Verification items for the finished model (mm, model axes). A direction names the side the tool comes from. Round coordinates to 2 decimals unless told otherwise and drop trailing zeros. Write each loop counter-clockwise with the first axis right and the second up, starting at its lowest first coordinate (ties: lowest second). Pieces come first, ordered by that corner, then holes. Notation, with made-up numbers: (12.5, -21) - (44.5, -21) arc R19 ccw to (44.5, 3) - close; hole circle Ø10 at (-35, -26). An arc over 180 degrees is marked (long way). Answer as a JSON object with one key per item and string values.
```python
from build123d import *

# Parameters (mm, degrees)
BOSS_EXTRUDE2_DEPTH           = 30
FILLET2_R                     = 10
FILLET3_R                     = 10
TAP_DRILL_FOR_M5_HELICOIL1_D  = 5.2
TAP_DRILL_FOR_M8_HELICOIL4_D  = 8.3
TAP_DRILL_FOR_M12_HELICOIL1_D = 12.5
TAP_DRILL_FOR_M8_TAP1_D       = 6.8
TAP_DRILL_FOR_M8_TAP1_DEPTH   = 25
TAP_DRILL_FOR_M8_TAP1_TIP     = 2.042926105
TAP_DRILL_FOR_M8_TAP2_D       = 6.8
TAP_DRILL_FOR_M8_TAP2_DEPTH   = 25
TAP_DRILL_FOR_M8_TAP2_TIP     = 2.042926105
TAP_DRILL_FOR_M8_TAP4_D       = 6.8
TAP_DRILL_FOR_M8_TAP4_DEPTH   = 25
TAP_DRILL_FOR_M8_TAP4_TIP     = 2.042926105
TAP_DRILL_FOR_M8_TAP5_D       = 6.8
TAP_DRILL_FOR_M8_TAP5_DEPTH   = 25
TAP_DRILL_FOR_M8_TAP5_TIP     = 2.042926105


with BuildPart() as part:
    # Sketch1 → Boss-Extrude2 (new body)
    with BuildSketch(Plane.XY):
        Polygon((0, 0), (370, 0), (370, 300), (185, 485), (0, 485), (0, 300), align=None)
        with BuildLine():
            Line((120, 323.710101352), (250, 323.710101352))
            ThreePointArc((250, 323.710101352), (273.710101352, 300), (250, 276.289898648))
            Line((250, 276.289898648), (120, 276.289898648))
            ThreePointArc((120, 276.289898648), (96.289898648, 300), (120, 323.710101352))
        make_face(mode=Mode.SUBTRACT)
    extrude(amount=BOSS_EXTRUDE2_DEPTH)

    # Fillet2
    fillet2_edges = [part.edges().sort_by_distance(p)[0] for p in [
        (370, 0, 15),
        (0, 0, 15),
    ]]
    fillet(fillet2_edges, radius=FILLET2_R)

    # Fillet3
    fillet3_edges = [part.edges().sort_by_distance(p)[0] for p in [
        (0, 485, 15),
        (185, 485, 15),
        (370, 300, 15),
    ]]
    fillet(fillet3_edges, radius=FILLET3_R)

    # Tap Drill for M5 Helicoil1 (through all)
    with Locations(Plane.XY.offset(30)):
        with Locations((300.970994454, 188.552878957), (181.155657642, 94.366491196), (100.424468133, 123.839782605), (151.041642508, 198.804458578), (260.6053997, 227.63702626), (283.030730119, 70.659713324), (88.89144106, 227.63702626), (165.137564486, 383.973615469), (315.707640159, 272.487687099), (61.981044557, 285.302161624)):
            Hole(TAP_DRILL_FOR_M5_HELICOIL1_D / 2)

    # Tap Drill for M8 Helicoil4 (through all)
    with Locations(Plane.XY.offset(30)):
        with Locations((65.825386914, 51.438001536), (45.322227674, 148.828007929), (236.898621828, 139.857875761), (241.383687912, 373.722035849), (338.132970578, 99.492281006), (223.443423576, 37.982803285), (193.970132168, 225.074131355), (36.992819232, 253.26597531)):
            Hole(TAP_DRILL_FOR_M8_HELICOIL4_D / 2)

    # Tap Drill for M12 Helicoil1 (through all)
    with Locations(Plane.XY.offset(30)):
        with Locations((163.856117033, 153.953797739), (325.318496053, 49.561393209), (128.616312088, 79.629845492), (189.485066084, 423.057762771), (110.676047753, 357.063218966), (97.220849501, 178.301299337), (325.318496053, 229.559197439), (53.19045969, 410.886687746)):
            Hole(TAP_DRILL_FOR_M12_HELICOIL1_D / 2)

    # Tap Drill for M8 Tap1
    with Locations(Plane(origin=(0, 0, 0), x_dir=(-1, 0, 0), z_dir=(0, -1, 0))):
        with Locations((-65, -15), (-315, -15)):
            Hole(TAP_DRILL_FOR_M8_TAP1_D / 2, depth=TAP_DRILL_FOR_M8_TAP1_DEPTH)
            with Locations((0, 0, -(TAP_DRILL_FOR_M8_TAP1_DEPTH + TAP_DRILL_FOR_M8_TAP1_TIP / 2))):  # 118° drill point
                Cone(0, TAP_DRILL_FOR_M8_TAP1_D / 2, TAP_DRILL_FOR_M8_TAP1_TIP, mode=Mode.SUBTRACT)

    # Tap Drill for M8 Tap2
    with Locations(Plane(origin=(335, 335, 0), x_dir=(0.7071067811865478, -0.7071067811865474, 0), z_dir=(0.7071067811865474, 0.7071067811865478, 0))):
        with Locations((-81.317279836, -15)):
            Hole(TAP_DRILL_FOR_M8_TAP2_D / 2, depth=TAP_DRILL_FOR_M8_TAP2_DEPTH)
            with Locations((0, 0, -(TAP_DRILL_FOR_M8_TAP2_DEPTH + TAP_DRILL_FOR_M8_TAP2_TIP / 2))):  # 118° drill point
                Cone(0, TAP_DRILL_FOR_M8_TAP2_D / 2, TAP_DRILL_FOR_M8_TAP2_TIP, mode=Mode.SUBTRACT)

    # Tap Drill for M8 Tap4
    with Locations(Plane(origin=(0, 485, 0), x_dir=(1, 0, 0), z_dir=(0, 1, 0))):
        with Locations((90, -15)):
            Hole(TAP_DRILL_FOR_M8_TAP4_D / 2, depth=TAP_DRILL_FOR_M8_TAP4_DEPTH)
            with Locations((0, 0, -(TAP_DRILL_FOR_M8_TAP4_DEPTH + TAP_DRILL_FOR_M8_TAP4_TIP / 2))):  # 118° drill point
                Cone(0, TAP_DRILL_FOR_M8_TAP4_D / 2, TAP_DRILL_FOR_M8_TAP4_TIP, mode=Mode.SUBTRACT)

    # Tap Drill for M8 Tap5
    with Locations(Plane(origin=(370, 0, 0), x_dir=(0, 0, -1), z_dir=(1, 0, 0))):
        with Locations((-15, 235.857864376), (-15, 70)):
            Hole(TAP_DRILL_FOR_M8_TAP5_D / 2, depth=TAP_DRILL_FOR_M8_TAP5_DEPTH)
            with Locations((0, 0, -(TAP_DRILL_FOR_M8_TAP5_DEPTH + TAP_DRILL_FOR_M8_TAP5_TIP / 2))):  # 118° drill point
                Cone(0, TAP_DRILL_FOR_M8_TAP5_D / 2, TAP_DRILL_FOR_M8_TAP5_TIP, mode=Mode.SUBTRACT)


solid = part.part
```
Q1. Material ranges on line 1 along X through (y, z) = (14.25, 15); line 2 along Y through (x, z) = (223.5, 9.25); line 3 along X through (y, z) = (224, 16.25), recorded low to high. Write a range as [from, to].
Geometry check:
{"line 1": "x = [0, 61.6], [68.4, 311.6], [318.4, 370]", "line 2": "y = [0, 33.83], [42.13, 276.29], [323.71, 446.5]", "line 3": "x = [0, 189.96], [197.98, 322.46], [328.17, 370]"}
Q2. Release check for a two-part mould opening along Z. For faces 3 (the flat face through (182, 246, 30)), 4 (the cylindrical face through (270.939, 381.136, 14.851)), 5 (the flat face through (97, 485, 15)) record: released by +Z, released by -Z, zero draft, split by the parting line, or undercut.
Geometry check:
{"face 3": "released by +Z", "face 4": "undercut", "face 5": "zero draft"}
Q3. Section check B-B, the plane z = 7. State how many separate pieces and enclosed holes the cut face has, then the cut area to 3 significant figures.
Geometry check:
{"separate pieces": "1", "enclosed holes": "27", "area": "153,000 mm2"}
Q4. Set-up check for faces 1 (the cylindrical face through (273.704, 300.521, 14.79)), 2 (the cylindrical face through (2.85, 481.99, 15.21)): record each of +Z, -Z, +X, -X, +Y, -Y from which the full face is reachable in a straight line by a thin tool's end or side.
Geometry check:
{"face 1": "+Z, -Z", "face 2": "+Z, -Z, -X, +Y"}
Q5. Section check A-A, the plane y = 310.5. Record the cut outline in (x, z).
Geometry check:
{"outline": "(0, 0) - (98.74, 0) - (98.74, 30) - (0, 30) - close; (271.26, 0) - (359.5, 0) - (359.5, 30) - (271.26, 30) - close"}
Q6. Gauge pin test, flat ends, axial feed: P1, Ø5.5, axis at x = 315, z = 15, coming from the +Y side; P2, Ø3, axis at x = 326.5, z = 16, coming from the +Y side. Record the tip position at first contact, or that the pin passes through.
Geometry check:
{"P1": "stops at y = 357.75", "P2": "stops at y = 345"}
